Geometry: see drawing. Coordinates: mm, zero at the bounding-box minimum. A direction names the side the tool comes from. Round coordinates to 2 decimals unless told otherwise and drop trailing zeros. Loops run counter-clockwise (first coordinate to the right, second up) from the corner with the lowest first, then second, coordinate; pieces in that order, holes last.
(1) Section A-A, the plane z = 3.25. Return the cut outline in (x, y).
(2) Section B-B, the plane y = 4. Return the cut outline in (x, z), plus the area to 3 significant figures.
(3) First-contact query: pin 1 Ø6 at (x, y) = (4.5, 23) entering from +Z; pin 2 Ø5 at (x, y) = (5, 27) entering from +Z. Flat tips, straight axial feed; report the tip coordinate or a pass-through.
(4) Section C-C, the plane x = 2.75. Return the cut outline in (y, z).
(5) Material intervals for probe 1 along X at (y, z) = (4.5, 8.5); probe 2 along Z at (x, y) = (6.25, 30), sorted ascending.
(6) Set-up query: the marked faces 4 and 5. Return all of +Z, -Z, +X, -X, +Y, -Y with unobstructed straight access to the full face (end or side cutting, diameter ignored); none if empty.
(7) Mould query, pull axis X, two halves, no side actions, for the marked faces 1, 2 and 3. Classes: pulls with the +X half, pulls with the -X half, needs draft (parallel to the pull), parting line crosses it, or undercut.
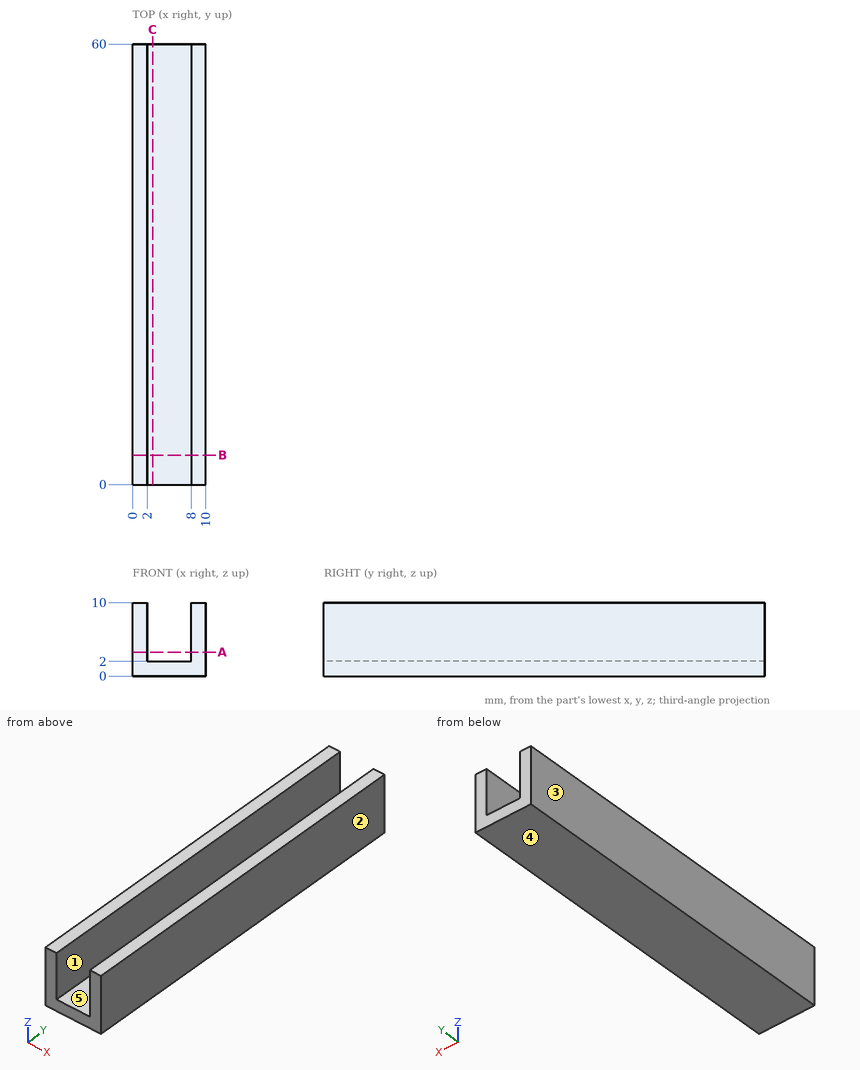
Output values:
1. outline: (0, 0) - (2, 0) - (2, 60) - (0, 60) - close; (8, 0) - (10, 0) - (10, 60) - (8, 60) - close
2. outline: (0, 0) - (10, 0) - (10, 10) - (8, 10) - (8, 2) - (2, 2) - (2, 10) - (0, 10) - close
2. area: 52.0 mm2
3. pin 1: stops at z = 10
3. pin 2: stops at z = 2
4. outline: (0, 0) - (60, 0) - (60, 2) - (0, 2) - close
5. probe 1: x = 0 to 2, 8 to 10
5. probe 2: z = 0 to 2
6. face 4: -Z, +X, -X, +Y, -Y
6. face 5: +Z, +Y, -Y
7. face 1: undercut
7. face 2: pulls with the +X half
7. face 3: pulls with the -X half
